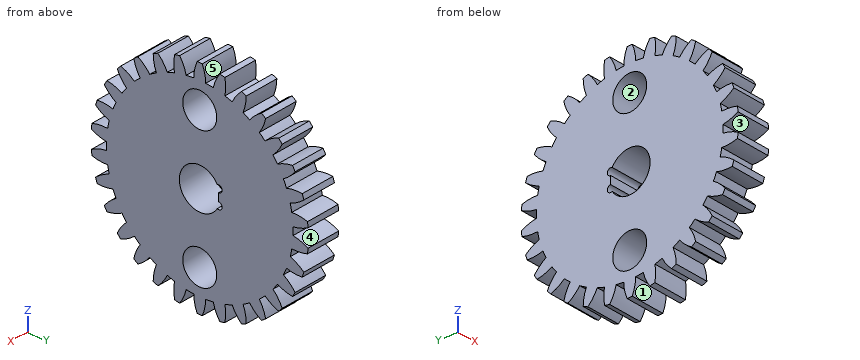
```python
from build123d import *

# Parameters (mm, degrees)
BASPROSKE_W         = 2.5
BASPROSKE_H         = 8
TOOTHCUT_DEPTH      = 12.586630226
TEETHCUTS_COUNT     = 30
TEETHCUTS_ANGLE     = 348
BORSKE_R            = 1.5
BORE_DEPTH          = 50.0000508
SKETCH_3_R          = 1.25
CUT_EXTRUDE_1_DEPTH = 12.568528524
EXTRUDE_1_DEPTH     = 2.5
SKETCH_5_R          = 0.25
CUT_EXTRUDE_2_DEPTH = 12.568528524


with BuildPart() as part:
    # BasProSke → Base-Revolve (revolve)
    with BuildSketch(Plane(origin=(0, 0, 0), x_dir=(1, 0, 0), z_dir=(0, 1, 0)), mode=Mode.PRIVATE) as base_revolve_sk:
        with Locations((1.25, 4)):
            Rectangle(BASPROSKE_W, BASPROSKE_H)
    revolve(base_revolve_sk.sketch.rotate(Axis((-10, 0, 0), (1, 0, 0)), 180), axis=Axis((-10, 0, 0), (1, 0, 0)))

    # TooCutSke → ToothCut (cut, through all)
    with BuildSketch(Plane(origin=(0, 0, 0), x_dir=(0, 0, -1), z_dir=(1, 0, 0))):
        with BuildLine():
            ThreePointArc((0.279013782, 6.868335119), (0, 6.874), (-0.279013782, 6.868335119))
            ThreePointArc((-0.279013782, 6.868335119), (-0.413500328, 7.452412324), (-0.661410108, 7.998098638))
            ThreePointArc((-0.661410108, 7.998098638), (0, 8.0254), (0.661410108, 7.998098638))
            ThreePointArc((0.661410108, 7.998098638), (0.413500328, 7.452412324), (0.279013782, 6.868335119))
        make_face()
    toothcut = extrude(amount=TOOTHCUT_DEPTH, mode=Mode.SUBTRACT)

    # TeethCuts: ToothCut ×30 about axis
    teethcuts_axis = Axis((-10, 0, 0), (1, 0, 0))
    for i in range(1, TEETHCUTS_COUNT):
        add(toothcut.rotate(teethcuts_axis, i * TEETHCUTS_ANGLE / (TEETHCUTS_COUNT - 1)), mode=Mode.SUBTRACT)

    # BorSke → Bore (cut, symmetric)
    with BuildSketch(Plane(origin=(0, 0, 0), x_dir=(0, 0, -1), z_dir=(1, 0, 0))):
        with Locations(Location((0, 0, 0), (0, 0, 180))):
            Circle(BORSKE_R)
    extrude(amount=BORE_DEPTH, both=True, mode=Mode.SUBTRACT)

    # 草图3 → 切除-拉伸1 (cut, through all)
    with BuildSketch(Plane.ZY):
        with Locations((-5, 0)):
            Circle(SKETCH_3_R)
        with Locations((5, 0)):
            Circle(SKETCH_3_R)
    extrude(amount=-CUT_EXTRUDE_1_DEPTH, mode=Mode.SUBTRACT)

    # 草图4 → 凸台-拉伸1 (add, through all)
    with BuildSketch(Plane.ZY):
        with BuildLine():
            Line((-0.538516481, 1.4), (0.538516481, 1.4))
            ThreePointArc((0.538516481, 1.4), (0, 1.5), (-0.538516481, 1.4))
        make_face()
    extrude(amount=-EXTRUDE_1_DEPTH)

    # 草图5 → 切除-拉伸2 (cut, through all)
    with BuildSketch(Plane.ZY):
        with Locations((-0.538516481, 1.4)):
            Circle(SKETCH_5_R)
        with Locations((0.538516481, 1.4)):
            Circle(SKETCH_5_R)
    extrude(amount=-CUT_EXTRUDE_2_DEPTH, mode=Mode.SUBTRACT)


solid = part.part
```
Part model, mm, in its own coordinate system. Face numbers are marked on the shaded views. A direction names the side the tool comes from. Coordinates: 2 decimals unless noted, no trailing zeros. Loops run counter-clockwise (first coordinate to the right, second up) from the corner with the lowest first, then second, coordinate; pieces in that order, holes last. Notation, with made-up numbers: (64.5, 11) - (86.5, 11) arc R19 ccw to (86.5, 34) - close; hole circle Ø8 at (54, 82.25). An arc over 180 degrees is marked (long way). Write item = value, one per line. Start each with the question number.
Item 1: Flat gauge pins, fed straight in: pin 1 Ø2 at (y, z) = (0, -5) entering from -X; pin 2 Ø0.5 at (x, z) = (1.5, 0) entering from -Y. Where does each tip first touch, or does it go through?
Item 2: Cut at B-B, the plane z = 0. Give the cut face in (x, y), and give its area (3 significant figures).
Item 3: Mould opens along Y. For the marked faces 3, 4 and 5 say: released by +Y, released by -Y, zero draft, split by the parting line, or undercut.
Item 4: 3-axis set-ups, long thin cutter, end or side, ignore diameter. For the marked faces 1 and 2: which of +Z, -Z, +X, -X, +Y, -Y reach the whole face in a straight line?
Item 5: Cut at A-A, the plane y = 0. Give the cut face in (x, z).
Item 6: Wall check: L1, parallel to Z at x = 2.4, y = 1.5; L2, parallel to Z at x = 1.15, y = 6; L3, parallel to Z at x = 0.4, y = -0.5. Give the ranges that are in metal, low to high. Write a range as from..to.
Item 7: Cut at C-C, the plane x = 1.3. State how many separate pieces and enclosed holes the cut face has, and give its area (3 significant figures).
The answers:
q1.pin_1 = through
q1.pin_2 = -6.87
q2.outline = (0, -6.87) - (2.5, -6.87) - (2.5, -1.5) - (0, -1.5) - close; (0, 1.4) - (2.5, 1.4) - (2.5, 6.87) - (0, 6.87) - close
q2.area = 27.1 mm2
q3.face_3 = released by -Y
q3.face_4 = released by +Y
q3.face_5 = undercut
q4.face_1 = -Z, +X, -X
q4.face_2 = +X, -X
q5.outline = (0, -8) - (2.5, -8) - (2.5, -6.25) - (0, -6.25) - close; (0, -3.75) - (2.5, -3.75) - (2.5, -1.5) - (0, -1.5) - close; (0, 1.5) - (2.5, 1.5) - (2.5, 3.75) - (0, 3.75) - close; (0, 6.25) - (2.5, 6.25) - (2.5, 8) - (0, 8) - close
q6.L1 = -7.86..-0.77, -0.31..0.31, 0.77..7.86
q6.L2 = -5.29..-5.07, -3.95..3.95, 5.07..5.29
q6.L3 = -6.86..-6.15, -3.85..-1.41, 1.41..3.85, 6.15..6.86
q7.separate_pieces = 1
q7.enclosed_holes = 3
q7.area = 155 mm2
